Could you check a few things on this model? Use its own coordinates, in mm. A direction names the side the tool comes from. Give positions to 0.01 mm unless a question says otherwise; leave off trailing zeros. Loops run counter-clockwise (first coordinate to the right, second up) from the corner with the lowest first, then second, coordinate; pieces in that order, holes last. Notation, with made-up numbers: (-20.5, 11) - (7.5, 11) arc R24 cw to (7.5, 24) - close; hole circle Ø6 at (10, -18). An arc over 180 degrees is marked (long way). One line per item, written item: value. Start each with the question number.
Q1. I want a section at D-D (z = -0.25). Please give me the cut outline in (x, y), then the cut area to 3 significant figures.
Q2. For faces 1 (the face through (-3.72, 0.74, -3.61)), 2 (the face through (3.72, 0.74, 3.61)), 3 (the face through (0, 2, -3.7)), 4 (the face through (0, 0, -4)), 5 (the face through (-3.61, 0.74, 3.72)), which set-ups out of +Z, -Z, +X, -X, +Y, -Y let a thin tool reach every point of the face, with its end or its side?
Q3. If we mould it in two halves opening along Z, with no side actions, what happens to faces 6 (the face through (3.61, 0.74, -3.72)), 7 (the face through (-6.18, 2.26, -5.13)), 8 (the face through (4, 1.5, 4))? For each: released by +Z, released by -Z, zero draft, split by the parting line, or undercut.
Q4. If I drill on line 1 (X direction, y = 1.75, z = 5.5); line 2 (X direction, y = 2.2, z = -5.08), over which ranges is the centre line in solid material (lowest first)? Write a range as from..to.
Q5. I want a section at B-B (z = 5.08). Please give me the cut outline in (x, y).
Q6. I want a section at C-C (x = 5.08). Please give me the cut outline in (y, z), then the cut area to 3 significant figures.
Q7. I want a section at A-A (y = 2.7). Please give me the cut outline in (x, z), then the cut area to 3 significant figures.
```python
from build123d import *

# Parameters (mm, degrees)
SKETCH_1_R               = 8.5
EXTRUDE_1_DEPTH          = 3
CUT_EXTRUDE_1_DEPTH      = 3
SKETCH_3_R               = 1.1
CUT_EXTRUDE_2_DEPTH      = 3
CUT_EXTRUDE_3_DEPTH      = 1.5
PATTERN_CIRCULAR_1_COUNT = 4


with BuildPart() as part:
    # 스케치1 → 보스-돌출1 (new body)
    with BuildSketch(Plane(origin=(0, 0, 0), x_dir=(1, 0, 0), z_dir=(0, 1, 0))):
        Circle(SKETCH_1_R)
    extrude(amount=EXTRUDE_1_DEPTH)

    # 스케치2 → 컷-돌출1 (cut)
    with BuildSketch(Plane(origin=(0, 3, 0), x_dir=(1, 0, 0), z_dir=(0, 1, 0))):
        with BuildLine():
            Line((-2.19089023, 3.7), (2.19089023, 3.7))
            ThreePointArc((2.19089023, 3.7), (0, -4.3), (-2.19089023, 3.7))
        make_face()
    extrude(amount=-CUT_EXTRUDE_1_DEPTH, mode=Mode.SUBTRACT)

    # 스케치3 → 컷-돌출2 (cut)
    with BuildSketch(Plane(origin=(0, 3, 0), x_dir=(1, 0, 0), z_dir=(0, 1, 0))):
        with Locations((5.08, 5.08)):
            Circle(SKETCH_3_R)
        with Locations((-5.08, -5.08)):
            Circle(SKETCH_3_R)
        with Locations((5.08, -5.08)):
            Circle(SKETCH_3_R)
        with Locations((-5.08, 5.08)):
            Circle(SKETCH_3_R)
    extrude(amount=-CUT_EXTRUDE_2_DEPTH, mode=Mode.SUBTRACT)

    # 스케치4 → 컷-돌출3 (cut)
    with BuildSketch(Plane.XZ):
        with BuildLine():
            Line((1.097301825, 8.4288747), (-8.4288747, -1.097301825))
            ThreePointArc((-8.4288747, -1.097301825), (-6.01040764, 6.01040764), (1.097301825, 8.4288747))
        make_face()
    cut_extrude_3 = extrude(amount=-CUT_EXTRUDE_3_DEPTH, mode=Mode.SUBTRACT)

    # 원형 패턴1: 컷-돌출3 ×4 about axis
    pattern_circular_1_axis = Axis((0, 0, 0), (0, 1, 0))
    for i in range(1, PATTERN_CIRCULAR_1_COUNT):
        add(cut_extrude_3.rotate(pattern_circular_1_axis, i * 360 / PATTERN_CIRCULAR_1_COUNT), mode=Mode.SUBTRACT)


solid = part.part
```
Worked answers:
1. outline: (-8.5, 1.5) - (-7.08, 1.5) - (-7.08, 0) - (-4.29, 0) - (-4.29, 3) - (-8.5, 3) - close; (4.29, 0) - (7.08, 0) - (7.08, 1.5) - (8.5, 1.5) - (8.5, 3) - (4.29, 3) - close
1. area: 21.0 mm²
2. face 1: -Z, -X, -Y
2. face 2: +Z, +X, -Y
2. face 3: +Y, -Y
2. face 4: +Z, -Z, +X, -X, -Y
2. face 5: +Z, -X, -Y
3. face 6: released by -Z
3. face 7: undercut
3. face 8: zero draft
4. line 1: x = -6.48..-6.1, -4.06..4.06, 6.1..6.48
4. line 2: x = -6.81..-6.18, -3.98..3.98, 6.18..6.81
5. outline: (-6.81, 1.5) - (-6.18, 1.5) - (-6.18, 3) - (-6.81, 3) - close; (-3.98, 1.5) - (-2.25, 1.5) - (-2.25, 0) - (2.25, 0) - (2.25, 1.5) - (3.98, 1.5) - (3.98, 3) - (-3.98, 3) - close; (6.18, 1.5) - (6.81, 1.5) - (6.81, 3) - (6.18, 3) - close
6. outline: (0, -2.25) - (1.5, -2.25) - (1.5, -3.98) - (3, -3.98) - (3, 3.98) - (1.5, 3.98) - (1.5, 2.25) - (0, 2.25) - close; (1.5, -6.81) - (3, -6.81) - (3, -6.18) - (1.5, -6.18) - close; (1.5, 6.18) - (3, 6.18) - (3, 6.81) - (1.5, 6.81) - close
6. area: 20.6 mm²
7. outline: circle Ø17 at (0, 0); hole circle Ø2.2 at (-5.08, -5.08); hole circle Ø2.2 at (-5.08, 5.08); hole (-2.19, -3.7) - (2.19, -3.7) arc R4.3 ccw (long way) to start; hole circle Ø2.2 at (5.08, -5.08); hole circle Ø2.2 at (5.08, 5.08)
7. area: 155 mm²
